from build123d import *

# Parameters (mm, degrees)
F0_R          = 13.005
F1_DEPTH      = 43
F2_R          = 7.75
F3_DEPTH      = 13.006
F3_DEPTH_BACK = 25
F4_W          = 7.1834153318
F4_H          = 12.5
F5_DEPTH      = 12.5
F6_T1_DEPTH   = 4.3042999791
F6_T3_DEPTH   = 20.2979349857
F6_T5_DEPTH   = 4.3042999791
F6_T8_ANGLE   = 97.7035470752
F6_T10_ANGLE  = 97.7035470752


# Not quite as in the source:
# - a fillet or chamfer that OpenCascade refuses, or shapes differently, is made with other operations: its cross-section is extruded or revolved along the edge and cut away or added


with BuildPart() as f1:
    # F0 (on Front) → F1 (new body)
    with BuildSketch(Plane.XZ):
        Circle(F0_R)
    extrude(amount=-F1_DEPTH)

    # F2 (on Right) → F3 (cut, two sides)
    with BuildSketch(Plane.YZ) as f3_sk:
        Circle(F2_R)
    extrude(amount=-F3_DEPTH, mode=Mode.SUBTRACT)
    extrude(f3_sk.sketch, amount=F3_DEPTH_BACK, mode=Mode.SUBTRACT)

    # F4 (on Top) → F5 (cut, symmetric)
    with BuildSketch(Plane.XY):
        with Locations((12.4917076659, 4.3530291878)):
            Rectangle(F4_W, F4_H)
        with Locations((-12.4917076659, 4.3530291878)):
            Rectangle(F4_W, F4_H)
    extrude(amount=F5_DEPTH, both=True, mode=Mode.SUBTRACT)

    # F6: chamfer of 0.5 on 8 edges, made by hand

    # F6_s2 → F6_t1 (cut)
    with BuildSketch(Plane.XY.offset(6.464158506)):
        Polygon((-8.4, 0), (-8.9, 0.5), (-8.9, 0), align=None)
        Polygon((8.9, 0.5), (8.4, 0), (8.9, 0), align=None)
    extrude(amount=F6_T1_DEPTH, mode=Mode.SUBTRACT)

    # F6_s4 → F6_t3 (cut)
    with BuildSketch(Plane.YZ.offset(-10.1489674928)):
        with BuildLine():
            Line((0, 8.234834546), (0.4696969697, 7.7357536644))
            ThreePointArc((0.4696969697, 7.7357536644), (0.2420339134, 7.7462196964), (0, 7.75))
            Line((0, 7.75), (0, 8.234834546))
        make_face()
        with BuildLine():
            Line((0, -8.234834546), (0.4696969697, -7.7357536644))
            ThreePointArc((0.4696969697, -7.7357536644), (0.2420339134, -7.7462196964), (0, -7.75))
            Line((0, -7.75), (0, -8.234834546))
        make_face()
    extrude(amount=F6_T3_DEPTH, mode=Mode.SUBTRACT)

    # F6_s6 → F6_t5 (cut)
    with BuildSketch(Plane.XY.offset(-10.7684584851)):
        Polygon((-8.9, 0.5), (-8.4, 0), (-8.9, 0), align=None)
        Polygon((8.9, 0.5), (8.4, 0), (8.9, 0), align=None)
    extrude(amount=F6_T5_DEPTH, mode=Mode.SUBTRACT)

    # F6_s7 → F6_t8 (revolve, cut)
    with BuildSketch(Plane(origin=(0, 0, 0), x_dir=(0, 1, 0), z_dir=(0.6580092951, 0, -0.7530098057))):
        Polygon((0.5, 13.005), (0, 12.505), (0, 13.005), align=None)
    revolve(axis=Axis((0, 0, 0), (0, -1, 0)), revolution_arc=F6_T8_ANGLE, mode=Mode.SUBTRACT)

    # F6_s9 → F6_t10 (revolve, cut)
    with BuildSketch(Plane(origin=(0, 0, 0), x_dir=(0, 1, 0), z_dir=(-0.6580092951, 0, 0.7530098057))):
        Polygon((0.5, 13.005), (0, 12.505), (0, 13.005), align=None)
    revolve(axis=Axis((0, 0, 0), (0, -1, 0)), revolution_arc=F6_T10_ANGLE, mode=Mode.SUBTRACT)


solid = f1.part
Here's how the part is built. I have some questions about the finished solid (model axes, mm). A direction names the side the tool comes from. Coordinates: 2 decimals unless noted, no trailing zeros. Loops run counter-clockwise (first coordinate to the right, second up) from the corner with the lowest first, then second, coordinate; pieces in that order, holes last.
1. Imagine slicing it at D-D, the plane y = 25. Please give me the cut outline in (x, z) (3 decimals), and give its area (3 significant figures).
2. Imagine slicing it at B-B, the plane z = 0. Please give me the cut outline in (x, y) (3 decimals), and give its area (3 significant figures).
3. For faces 1 (the flat face through (0, 0, 10)), 2 (the flat face through (8.9, 9, 0)), 3 (the flat face through (-8.9, 9, 0)), which set-ups out of +Z, -Z, +X, -X, +Y, -Y let a thin tool reach every point of the face, with its end or its side?
4. I need wall thicknesses on L1, parallel to Y at x = -10.75, z = 6.25; L2, parallel to Z at x = -0.75, y = 7; L3, parallel to Z at x = -2.5, y = 29. Which ranges of each line are inside material? Lowest first, please.
5. Imagine slicing it at C-C, the plane y = 3.5. Please give me the cut outline in (x, z) (3 decimals), and give its area (3 significant figures).
6. If we mould it in two halves opening along Z, with no side actions, what happens to faces 4 (the cylindrical face through (12.013, 21.452, -4.981)), 5 (the conical face through (-0.133, 0.135, -12.64)), 6 (the flat face through (0, 0, -10)), 7 (the cylindrical face through (0.12, 7.75, -0.16))? For each: pulls with the +Z half, pulls with the -Z half, needs draft (parallel to the pull), parting line crosses it, or undercut.
7. Imagine slicing it at A-A, the plane x = 0. Please give me the cut outline in (y, z) (3 decimals), and give its area (3 significant figures).
8. For P1, Ø5, axis at y = 5.5, z = 10.5, coming from the +X side; P2, Ø3, axis at x = -6, y = 5.5, coming from the +Z side; P3, Ø4.5, axis at x = 11.5, z = 1, coming from the -Y side, each with a flat end and sliding along its axis, tell me the tip position at first contact or that it passes through.
Taken from the geometry:
1. outline: circle Ø26.01 at (0, 0)
1. area: 531 mm2
2. outline: (-13.005, 10.603) - (-8.9, 10.603) - (-8.9, 7.75) - (8.9, 7.75) - (8.9, 10.603) - (13.005, 10.603) - (13.005, 43) - (-13.005, 43) - close
2. area: 893 mm2
3. face 1: +Z, -Z, +X, -X, -Y
3. face 2: +Z, -Z, +X, -Y
3. face 3: +Z, -Z, -X, -Y
4. L1: y = 10.6 to 43
4. L2: z = -12.98 to -3.33, 3.33 to 12.98
4. L3: z = -12.76 to 12.76
5. outline: (-8.9, -9.483) arc R13.005 ccw to (8.9, -9.483) - (8.9, -6.915) - (-8.9, -6.915) - close; (-8.9, 6.915) - (8.9, 6.915) - (8.9, 9.483) arc R13.005 ccw to (-8.9, 9.483) - close
5. area: 178 mm2
6. face 4: parting line crosses it
6. face 5: pulls with the -Z half
6. face 6: needs draft
6. face 7: undercut
7. outline: (0, -12.505) - (0.5, -13.005) - (43, -13.005) - (43, 13.005) - (0.5, 13.005) - (0, 12.505) - (0, 8.235) - (0.47, 7.736) arc R7.75 cw to (0.47, -7.736) - (0, -8.235) - close
7. area: 1,020 mm2
8. P1: stops at x = 8.9
8. P2: stops at z = 12.2
8. P3: stops at y = 10.6
